Autodesk Inventor part; units mm, degrees
ref_plane "YZ Plane" through (0, 0, 0) normal (1, 0, 0) x (0, 1, 0)
ref_plane "XZ Plane" through (0, 0, 0) normal (0, 1, 0) x (-1, 0, 0)
ref_plane "XY Plane" through (0, 0, 0) normal (0, 0, 1) x (1, 0, 0)
sketch "草图1" plane through (0, 0, 0) normal (0, 0, 1) x (1, 0, 0)
  line L0 (-31.2, 0) -> (5.2, 0) construction
  line L1 (0, -36.4) -> (0, 36.4) construction
  line L2 (-26, 22.5) -> (-13, 22.5)
  line L3 (-13, -22.5) -> (-26, -22.5)
  line L4 (-26, -22.5) -> (-26, 22.5)
  line L5 (-13, 26) -> (0, 26)
  line L6 (0, 26) -> (0, -26)
  line L7 (0, -26) -> (-13, -26)
  line L8 (-13, -26) -> (-13, -22.5)
  line L9 (-13, 22.5) -> (-13, 26)
  line L10 (-26, 20) -> (0, 20)
  line L11 (0, 20) -> (0, -20)
  line L12 (0, -20) -> (-26, -20)
  line L13 (-26, -20) -> (-26, 20)
  point P0 (0, 0)
  point P1 (0, 20)
  dimension "d0" = 26
  dimension "d1" = 13
  dimension "d2" = 45
  dimension "d3" = 52
  dimension "d4" = 40
revolve "旋转1" add sketch "草图1" angle 360 about axis through (-10, 0, 0) along (1, 0, 0) contours L2 L9 L5 L6 L10 L4
sketch "草图2" plane through (0, 0, 0) normal (0, 0, 1) x (1, 0, 0)
  line L0 (-26, -22.5) -> (-26, 22.5) construction
  line L1 (-13, -22.5) -> (-13, 22.5) construction
  line L2 (-26, 22.5) -> (-13, 22.5) construction
  line L3 (-26, -22.5) -> (-13, -22.5) construction
  line L4 (-21, 39.5) -> (-13, 39.5)
  line L5 (-13, 39.5) -> (-13, -39.5)
  line L6 (-13, -39.5) -> (-21, -39.5)
  line L7 (-21, -39.5) -> (-21, 39.5)
  line L8 (-81.7478, 0) -> (13.6246, 0) construction
  line L9 (-21, 22.5) -> (-13, 22.5)
  line L10 (-21, 39.5) -> (-20, 37.7679)
  line L11 (-20, 37.7679) -> (-19, 39.5)
  line L12 (-19, 39.5) -> (-18, 37.7679)
  line L13 (-18, 37.7679) -> (-17, 39.5)
  line L14 (-17, 39.5) -> (-16, 37.7679)
  line L15 (-16, 37.7679) -> (-15, 39.5)
  line L16 (-15, 39.5) -> (-14, 37.7679)
  line L17 (-14, 37.7679) -> (-13, 39.5)
  point P0 (0, 0)
  dimension "d6" = 8
  dimension "d7" = 79
  dimension "d8" = 60
  dimension "d9" = 2
  dimension "d10" = 2
revolve "旋转2" add sketch "草图2" angle 360 about axis through (-10, 0, 0) along (1, 0, 0) contours L10 L11 L12 L13 L14 L15 L16 L17 L5 L9 L7
properties part number "轴套1"
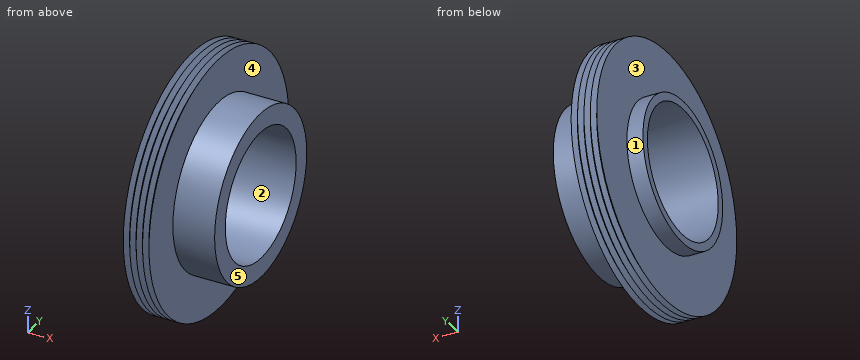
Build history of the part. All positions in model axes, mm. Face numbers are marked on the shaded views. A direction names the side the tool comes from. Give positions to 0.01 mm unless a question says otherwise; leave off trailing zeros. Loops run counter-clockwise (first coordinate to the right, second up) from the corner with the lowest first, then second, coordinate; pieces in that order, holes last. Notation, with made-up numbers: (55, 27) - (75, 27) arc R30 ccw to (75, 54) - close; hole circle Ø2 at (-34, 70.25). An arc over 180 degrees is marked (long way). Use a Markdown table: item, result.
(1) Which spindle directions (+Z, -Z, +X, -X, +Y, -Y) get a long thin tool onto all of the face, cutting with end or side? Do the marked faces 4 and 5. Say none if no direction does.
Taken from the geometry:
| item | result |
|---|---|
| face 4 | +X |
| face 5 | +Z, -Z, +X, +Y, -Y |
(2) Band-saw the part on A-A (x = -7). Give the cut face in (y, z), and give its area (3 significant figures).
Taken from the geometry:
| item | result |
|---|---|
| outline | circle Ø52 at (0, 0); hole circle Ø40 at (0, 0) |
| area | 867 mm2 |
(3) Wall check: line 1 along X through (y, z) = (-19.5, -32.5); line 2 along Z through (x, y) = (-11.75, 0); line 3 along Z through (x, y) = (-5.75, 6.5). Give the ranges that are in metal, low to high.
Taken from the geometry:
| item | result |
|---|---|
| line 1 | -21 to -20.08, -19.92 to -18.08, -17.92 to -16.08, -15.92 to -14.08, -13.92 to -13 |
| line 2 | -26 to -20, 20 to 26 |
| line 3 | -25.17 to -18.91, 18.91 to 25.17 |
(4) Pull direction Y, two halves, no side cores. Call the marked faces 1, 2 and 3: +Y half, -Y half, draft (parallel to the pull), parting line (faces both ways), or undercut.
Taken from the geometry:
| item | result |
|---|---|
| face 1 | parting line |
| face 2 | undercut |
| face 3 | draft |
(5) Drop flat-ended pins along their axis: pin 1 Ø2 at (x, y) = (-14, 22) entering from -Z; pin 2 Ø1.5 at (x, y) = (-21, 19) entering from +Z; pin 3 Ø4 at (x, z) = (-11.5, -23) entering from -Y; pin 4 Ø6 at (x, z) = (-2.5, 30) entering from +Y. Give the stop position or say it passes through.
Taken from the geometry:
| item | result |
|---|---|
| pin 1 | z = -32.91 |
| pin 2 | z = 35.03 |
| pin 3 | y = -33.02 |
| pin 4 | through |
